from build123d import *

# Parameters (mm, degrees)
BOSS_EXTRUDE1_DEPTH = 5
BOSS_EXTRUDE2_DEPTH = 15
FILLET1_R           = 2


with BuildPart() as part:
    # Sketch1 → Boss-Extrude1 (new body)
    with BuildSketch(Plane(origin=(0, 0, 0), x_dir=(1, 0, 0), z_dir=(0, 1, 0))):
        Polygon((71.24355653, 70), (-71.24355653, 70), (-90, 0), (90, 0), align=None)
    extrude(amount=BOSS_EXTRUDE1_DEPTH)

    # Sketch2 → Boss-Extrude2 (add)
    with BuildSketch(Plane(origin=(0, 5, 0), x_dir=(1, 0, 0), z_dir=(0, 1, 0))):
        Polygon((68.941575566, 67), (-68.941575566, 67), (-86.894171459, 0), (-90, 0), (-71.24355653, 70), (71.24355653, 70), (90, 0), (86.894171459, 0), align=None)
    extrude(amount=BOSS_EXTRUDE2_DEPTH)

    # Fillet1
    fillet1_edges = [part.edges().sort_by_distance(p)[0] for p in [
        (-68.941575566, 12.5, -67),
        (68.941575566, 12.5, -67),
        (-71.24355653, 10, -70),
        (71.24355653, 10, -70),
    ]]
    fillet(fillet1_edges, radius=FILLET1_R)


solid = part.part
Verification items for the finished model (mm, model axes). A direction names the side the tool comes from. Give positions to 0.01 mm unless a question says otherwise; leave off trailing zeros. Write each loop counter-clockwise with the first axis right and the second up, starting at its lowest first coordinate (ties: lowest second). Pieces come first, ordered by that corner, then holes.
(1) Cross-section at D-D (y = 2.5). Enter the section's corners in (x, z), plus the area to 3 significant figures.
(2) Material ranges on line 1 (Y direction, x = -38, z = -44); line 2 (X direction, y = 17.5, z = -19); line 3 (X direction, y = 14, z = -41.5), recorded low to high.
(3) Cross-section at B-B (x = -55). Enter the section's corners in (y, z).
(4) Access from +Z, -Z, +X, -X, +Y, -Y to the whole of each face (thin tool, end or side, straight path). Record for faces 4 (the face through (-1, 0, -35)), 5 (the face through (78.24, 12.4, -32.3)).
(5) Mould release check, pull along X, two halves, no side actions. Record for faces 1 (the face through (-80.95, 9.86, -33.78)), 2 (the face through (-78, 12.4, -33.2)), 3 (the face through (80.69, 9.86, -34.74)): +X half, -X half, draft (parallel to the pull), parting line (faces both ways), or undercut.
(6) Gauge pin test, flat ends, axial feed: pin 1 (5 mm diameter, centred on y = 12, z = -11, fed in from +X); pin 2 (7.5 mm diameter, centred on x = -28.5, y = 14, fed in from +Z); pin 3 (4 mm diameter, centred on y = 13, z = -45.5, fed in from +X); pin 4 (1 mm diameter, centred on x = -47, z = -24, fed in from -Y). Record the tip position at first contact, or that the pin passes through.
(7) Cross-section at C-C (z = -33). Enter the section's corners in (x, y), plus the area to 3 significant figures.
(8) Cross-section at A-A (y = 10). Enter the section's corners in (x, z), plus the area to 3 significant figures.
Worked out:
1. outline: (-90, 0) - (-71.64, -68.52) arc R2 ccw to (-69.71, -70) - (69.71, -70) arc R2 ccw to (71.64, -68.52) - (90, 0) - close
1. area: 11,300 mm2
2. line 1: y = 0 to 5
2. line 2: x = -84.91 to -81.8, 81.8 to 84.91
2. line 3: x = -78.88 to -75.77, 75.77 to 78.88
3. outline: (0, -70) - (20, -70) - (20, -67) - (5, -67) - (5, 0) - (0, 0) - close
4. face 4: +Z, -Z, +X, -X, -Y
4. face 5: +Z, +Y
5. face 1: -X half
5. face 2: undercut
5. face 3: +X half
6. pin 1: stops at x = 87.72
6. pin 2: stops at z = -67
6. pin 3: stops at x = 78.34
6. pin 4: stops at y = 0
7. outline: (-81.16, 0) - (81.16, 0) - (81.16, 20) - (78.05, 20) - (78.05, 5) - (-78.05, 5) - (-78.05, 20) - (-81.16, 20) - close
7. area: 905 mm2
8. outline: (-90, 0) - (-71.64, -68.52) arc R2 ccw to (-69.71, -70) - (69.71, -70) arc R2 ccw to (71.64, -68.52) - (90, 0) - (86.89, 0) - (69.34, -65.52) arc R2 cw to (67.41, -67) - (-67.41, -67) arc R2 cw to (-69.34, -65.52) - (-86.89, 0) - close
8. area: 846 mm2
